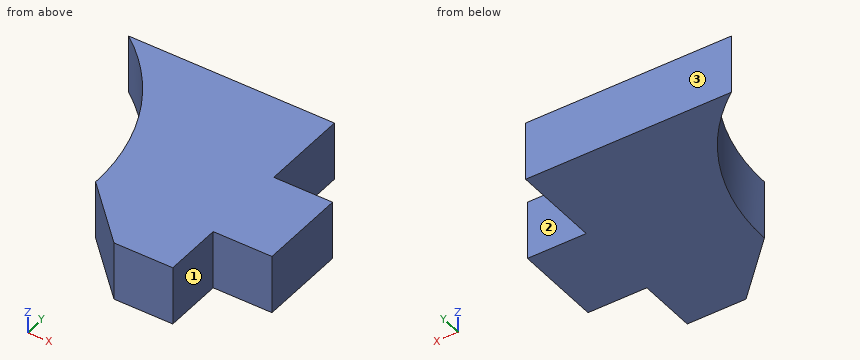
from build123d import *

# Parameters (mm, degrees)
BOSS_EXTRUDE1_DEPTH = 3


with BuildPart() as part:
    # Sketch1 → Boss-Extrude1 (new body)
    with BuildSketch(Plane.XY):
        with BuildLine():
            Line((490.924864814, 8.749554885), (490.924864814, 5.749554885))
            Line((490.924864814, 5.749554885), (487.924864814, 5.749554885))
            Line((487.924864814, 5.749554885), (484.924864814, 8.749554885))
            ThreePointArc((484.924864814, 8.749554885), (483.737170712, 13.780707835), (480.424864814, 17.749554885))
            Line((480.424864814, 17.749554885), (490.924864814, 17.749554885))
            Line((490.924864814, 17.749554885), (490.924864814, 13.249554885))
            Line((490.924864814, 13.249554885), (493.924864814, 13.249554885))
            Line((493.924864814, 13.249554885), (493.924864814, 8.749554885))
            Line((493.924864814, 8.749554885), (490.924864814, 8.749554885))
        make_face()
    extrude(amount=BOSS_EXTRUDE1_DEPTH)


solid = part.part
Verification items for the finished model (mm, model axes). Face numbers are marked on the shaded views. A direction names the side the tool comes from. Give positions to 0.01 mm unless a question says otherwise; leave off trailing zeros. Loops run counter-clockwise (first coordinate to the right, second up) from the corner with the lowest first, then second, coordinate; pieces in that order, holes last. Notation, with made-up numbers: (36, 84) - (55, 84) arc R11 cw to (55, 100) - close; hole circle Ø8 at (46.25, -21.5). An arc over 180 degrees is marked (long way). Write item = value, one per line. Start each with the question number.
Q1. Depth check by flat-ended pin: P1, Ø0.9, axis at x = 492.5, z = 2, coming from the +Y side; P2, Ø0.9, axis at y = 6.5, z = 1, coming from the +X side; P3, Ø1, axis at y = 16.5, z = 2.5, coming from the -X side. Enter the tip coordinate at first touch or a pass-through.
Q2. Cross-section at B-B, the plane x = 491.5. Enter the section's corners in (y, z).
Q3. Cross-section at C-C, the plane y = 10.5. Enter the section's corners in (x, z), and give its area (3 significant figures).
Q4. Tool access check on the marked faces 1, 2 and 3. Record the directions out of +Z, -Z, +X, -X, +Y, -Y that give a thin tool (end or side, any length) a straight path to the whole face; none if there is none.
Q5. Thickness scan on line 1 (Y direction, x = 491.75, z = 2.4); line 2 (X direction, y = 12.5, z = 2); line 3 (X direction, y = 7.25, z = 2.75). Record the ranges inside material, lowest first.
Q6. Cross-section at A-A, the plane z = 2.2. Enter the section's corners in (x, y).
Answer key:
q1.P1 = 13.25
q1.P2 = 490.92
q1.P3 = 481.32
q2.outline = (8.75, 0) - (13.25, 0) - (13.25, 3) - (8.75, 3) - close
q3.outline = (484.79, 0) - (493.92, 0) - (493.92, 3) - (484.79, 3) - close
q3.area = 27.4 mm^2
q4.face_1 = +Z, -Z, +X, -Y
q4.face_2 = +Z, -Z, +X, +Y
q4.face_3 = +Z, -Z, +X, -X, +Y
q5.line_1 = 8.75 to 13.25
q5.line_2 = 484.28 to 493.92
q5.line_3 = 486.42 to 490.92
q6.outline = (480.42, 17.75) arc R11.25 cw to (484.92, 8.75) - (487.92, 5.75) - (490.92, 5.75) - (490.92, 8.75) - (493.92, 8.75) - (493.92, 13.25) - (490.92, 13.25) - (490.92, 17.75) - close
